Model file for the job. Use its own axes, mm. A direction names the side the tool comes from. Give positions to 0.01 mm unless a question says otherwise; leave off trailing zeros. Order: outer loops, then holes, each group sorted by start corner. A loop starts at its lowest first (then second) coordinate and runs counter-clockwise, first axis right, second up. Notation, with made-up numbers: M -6,61 L 47,61 A23 ccw 47,88 Z; hole C 14.5,66.25 d8. An arc over 180 degrees is marked long. Return JSON: item names as keys, results as strings. Group by question number.
1. Slice it at A-A on x = 6. List the corners of the cut face in (y, z).
2. Two-plate mould, pull along Z, no slides. Class faces 1 (the face through (6, 15, 35)), 2 (the face through (-21.76, 12.41, -8.17)), 3 (the face through (13, 30, 7)): released by +Z, released by -Z, zero draft, split by the parting line, or undercut.
3. Pin check, flat tips, straight feed: pin 1 (2 mm diameter, centred on y = 21.5, z = -22.5, fed in from +X); pin 2 (10.5 mm diameter, centred on y = 15, z = 31.5, fed in from +X); pin 3 (7.5 mm diameter, centred on y = 15, z = -4.8, fed in from +X); pin 4 (2 mm diameter, centred on x = 22, y = 15, fed in from -Z). Stop position of each tip, or through.
4. Slice it at C-C on y = 24. List the corners of the cut face in (x, z), then the cut area to 3 significant figures.
5. 3-axis set-ups, long thin cutter, end or side, ignore diameter. For faces 4 (the face through (-10, 11, 31)), 5 (the face through (-0.2, 14.8, -36.5)), 6 (the face through (-15.933, 14.79, -0.211)): which of +Z, -Z, +X, -X, +Y, -Y reach the whole face in a straight line?
6. Wall check: probe 1 along X at (y, z) = (14, 18); probe 2 along Y at (x, z) = (6, 31.5); probe 3 along Z at (x, y) = (-3.5, 18). Give the ranges that are in metal, low to high. Write a range as [from, to].
7. Slice it at B-B on z = 31.5. List the corners of the cut face in (x, y), then the cut area to 4 significant figures.
8. Slice it at D-D on x = 12.5. List the corners of the cut face in (y, z).
from build123d import *

# Parameters (mm, degrees)
BOSS_EXTRUDE2_DEPTH = 30
SKETCH2_R           = 4.25
CUT_EXTRUDE1_DEPTH  = 55.999999228
SKETCH5_R           = 3.25
CUT_EXTRUDE2_DEPTH  = 30


with BuildPart() as part:
    # Sketch1 → Boss-Extrude2 (new body)
    with BuildSketch(Plane(origin=(0, 0, 0), x_dir=(1, 0, 0), z_dir=(0, 1, 0))):
        with BuildLine():
            Line((-1.499999614, -22.769695991), (-1.499999614, -34.999999869))
            Line((-1.499999614, -34.999999869), (-9.999999614, -34.999999869))
            Line((-9.999999614, -34.999999869), (-9.999999614, -26.999999869))
            Line((-9.999999614, -26.999999869), (-27.499999614, -2.699999869))
            Line((-27.499999614, -2.699999869), (-27.499999614, 12.300000131))
            Line((-27.499999614, 12.300000131), (-14.093884058, 29.689647964))
            ThreePointArc((-14.093884058, 29.689647964), (0, 36.500000672), (14.093884058, 29.689647964))
            Line((14.093884058, 29.689647964), (27.499999614, 12.300000131))
            Line((27.499999614, 12.300000131), (27.499999614, -2.699999869))
            Line((27.499999614, -2.699999869), (9.999999344, -26.999999675))
            Line((9.999999344, -26.999999675), (9.999999344, -34.999999869))
            Line((9.999999344, -34.999999869), (1.500000386, -34.999999869))
            Line((1.500000386, -34.999999869), (1.500000386, -22.769695748))
            ThreePointArc((1.500000386, -22.769695748), (4.0311289, -20.958039634), (4.999999869, -18))
            Line((4.999999869, -18), (4.999999869, -11.224185235))
            ThreePointArc((4.999999869, -11.224185235), (16.5, 4.5), (4.999999869, 20.224185235))
            Line((4.999999869, 20.224185235), (4.999999869, 27))
            ThreePointArc((4.999999869, 27), (0, 31.999999869), (-4.999999869, 27))
            Line((-4.999999869, 27), (-4.999999869, 20.224185235))
            ThreePointArc((-4.999999869, 20.224185235), (-16.5, 4.5), (-4.999999869, -11.224185235))
            Line((-4.999999869, -11.224185235), (-4.999999869, -18))
            ThreePointArc((-4.999999869, -18), (-4.031128661, -20.95803996), (-1.499999614, -22.769695991))
        make_face()
    extrude(amount=BOSS_EXTRUDE2_DEPTH)

    # Sketch2 → Cut-Extrude1 (cut, through all)
    with BuildSketch(Plane.ZY.offset(27.499999614)):
        with Locations((-4.800000131, 15)):
            Circle(SKETCH2_R)
    extrude(amount=-CUT_EXTRUDE1_DEPTH, mode=Mode.SUBTRACT)

    # Sketch5 → Cut-Extrude2 (cut)
    with BuildSketch(Plane.ZY.offset(9.999999614)):
        with Locations((31.499999869, 15)):
            Circle(SKETCH5_R)
    extrude(amount=-CUT_EXTRUDE2_DEPTH, mode=Mode.SUBTRACT)


solid = part.part
Result:
{
 "1": {"outline": "M 0,-35.47 L 30,-35.47 L 30,-19.87 L 0,-19.87 Z; M 0,10.87 L 30,10.87 L 30,35 L 0,35 Z; hole C 15,31.5 d6.5"},
 "2": {"face 1": "released by +Z", "face 2": "undercut", "face 3": "zero draft"},
 "3": {"pin 1": "stops at x = 20.41", "pin 2": "stops at x = 10.54", "pin 3": "passes through", "pin 4": "stops at z = -20.73"},
 "4": {"outline": "M -27.5,-12.3 L -14.09,-29.69 A17.99 ccw 14.09,-29.69 L 27.5,-12.3 L 27.5,2.7 L 10,27 L 10,35 L 1.5,35 L 1.5,22.77 A5 cw 5,18 L 5,11.22 A16.5 cw 5,-20.22 L 5,-27 A5 cw -5,-27 L -5,-20.22 A16.5 cw -5,11.22 L -5,18 A5 cw -1.5,22.77 L -1.5,35 L -10,35 L -10,27 L -27.5,2.7 Z", "area": "1,660 mm2"},
 "5": {"face 4": "+Z, -X, +Y, -Y", "face 5": "-Z, +Y, -Y", "face 6": "+Y, -Y"},
 "6": {"probe 1": "x = [-16.48, -5], [5, 16.48]", "probe 2": "y = [0, 11.75], [18.25, 30]", "probe 3": "z = [-36.16, -30.57], [21.57, 30.25], [32.75, 35]"},
 "7": {"outline": "M -10,0 L -1.5,0 L -1.5,11.75 L -10,11.75 Z; M -10,18.25 L -1.5,18.25 L -1.5,30 L -10,30 Z; M 1.5,0 L 10,0 L 10,11.75 L 1.5,11.75 Z; M 1.5,18.25 L 10,18.25 L 10,30 L 1.5,30 Z", "area": "399.5 mm2"},
 "8": {"outline": "M 0,-31.45 L 30,-31.45 L 30,-15.27 L 0,-15.27 Z; M 0,6.27 L 30,6.27 L 30,23.53 L 0,23.53 Z"}
}
